Autodesk Inventor part; units mm, degrees
ref_plane "YZ Plane" through (0, 0, 0) normal (1, 0, 0) x (0, 1, 0)
ref_plane "XZ Plane" through (0, 0, 0) normal (0, 1, 0) x (-1, 0, 0)
ref_plane "XY Plane" through (0, 0, 0) normal (0, 0, 1) x (1, 0, 0)
ref_plane "Work Plane1" through (0, 0, 0) normal (0, 0, 1) x (1, 0, 0)
sketch "Sketch1" plane through (0, 0, 0) normal (0, 0, 1) x (1, 0, 0)
  circle A0 centre (114.3836, 12.2466) radius 10
  circle A1 centre (114.3836, 12.2466) radius 10
  line L0 (114.3836, 12.2466) -> (76.8836, 12.2466)
  line L1 (124.7866, -536.2038) -> (-25.2134, -536.2038)
  line L2 (114.3836, 12.2466) -> (114.3836, -536.2038)
  line L3 (76.8836, 12.2466) -> (76.8836, 52.1676)
  line L4 (76.8836, 52.1676) -> (226.8836, 52.1676)
  line L5 (226.8836, 52.1676) -> (226.8836, -17.8324)
  line L6 (226.8836, -17.8324) -> (76.8836, -17.8324)
  line L7 (76.8836, -17.8324) -> (76.8836, 12.2466)
  circle A2 centre (114.3836, 12.2466) radius 10
  line L8 (151.8836, 52.1676) -> (151.8836, -17.8324)
  circle A3 centre (189.3836, 12.2466) radius 10
  line L9 (76.8836, 52.1676) -> (76.8836, 42.1676)
  line L10 (76.8836, 42.1676) -> (226.8836, 42.1676)
  line L11 (226.8836, 52.1676) -> (76.8836, 52.1676)
  line L12 (76.8836, 52.1676) -> (76.8836, 42.1676)
  line L13 (76.8836, 42.1676) -> (226.8836, 42.1676)
  line L14 (226.8836, 42.1676) -> (226.8836, 52.1676)
  point P0 (0, 0)
  dimension "d0" = 37.5
  dimension "d1" = 548.4504
  dimension "d2" = 39.921
  dimension "d3" = 150
  dimension "d4" = 70
  dimension "d5" = 10
  dimension "d6" = 150
extrude "Extrusion1" add sketch "Sketch1" along normal blind 5 contours A0 L0 L3 L10 L8 L6 L2 | A0 L2 L6 L7 L0 | L3 L4 L8 L10 | L8 L10 L5 L6 | L8 L4 L5 L10
sketch "Sketch3" plane through (0, 0, 0) normal (0, 0, -1) x (-1, 0, 0)
  line L0 (-226.8836, 52.1676) -> (-76.8836, 52.1676)
  line L1 (-76.8836, 42.1676) -> (-226.8836, 42.1676)
  line L2 (-226.8836, 52.1676) -> (-76.8836, 52.1676)
  line L3 (-76.8836, 52.1676) -> (-76.8836, 42.1676)
  line L4 (-76.8836, 42.1676) -> (-226.8836, 42.1676)
  line L5 (-226.8836, 42.1676) -> (-226.8836, 52.1676)
  point P0 (0, 0)
extrude "Extrusion2" add sketch "Sketch3" along normal blind 80
sketch "Sketch4" plane through (0, 0, -80) normal (0, 0, -1) x (-1, 0, 0)
  line L0 (-226.8836, 52.1676) -> (-76.8836, 52.1676)
  line L1 (-76.8836, -17.8324) -> (-226.8836, -17.8324)
  line L2 (-226.8836, 52.1676) -> (-76.8836, 52.1676)
  line L3 (-76.8836, 52.1676) -> (-76.8836, -17.8324)
  line L4 (-76.8836, -17.8324) -> (-226.8836, -17.8324)
  line L5 (-226.8836, -17.8324) -> (-226.8836, 52.1676)
  point P0 (0, 0)
  point P1 (-76.8836, 52.1676)
extrude "Extrusion3" add sketch "Sketch4" along normal blind 5
sketch "Sketch6" plane through (0, 0, -85) normal (0, 0, -1) x (-1, 0, 0)
  line L0 (-98.3957, 24.2628) -> (62.6208, -189.9747)
  arc A0 (-98.3957, 24.2628) -> (-130.3715, 0.2304) centre (-114.3836, 12.2466) ccw
  line L1 (30.6451, -214.007) -> (-130.3715, 0.2304)
  arc A1 (30.6451, -214.007) -> (62.6208, -189.9747) centre (46.6329, -201.9908) ccw
  circle A2 centre (46.6329, -201.9908) radius 9.25
  circle A3 centre (-114.3836, 12.2466) radius 10
  circle A4 centre (-189.3836, 12.2466) radius 10
  point P0 (0, 0)
extrude "Extrusion4" cut sketch "Sketch6" against normal blind 10 contours A3 | A4
sketch "Sketch8" plane through (76.8836, 52.1676, 5) normal (0, 1, 0) x (1, 0, 0)
  line L0 (0, 0) -> (0, 90)
  line L1 (150, 0) -> (0, 0)
  line L2 (150, 90) -> (150, 0)
  line L3 (0, 90) -> (150, 90)
  point P0 (-76.8836, 5)
extrude "Extrusion6" add sketch "Sketch8" along normal blind 0.079
properties part number "korona"
Geometry: final body of the model. Coordinates: model frame, mm. A direction names the side the tool comes from. Round coordinates to 2 decimals unless told otherwise and drop trailing zeros. Write each loop counter-clockwise with the first axis right and the second up, starting at its lowest first coordinate (ties: lowest second). Pieces come first, ordered by that corner, then holes.
Item 1: Section query A-A (y = -4). Return loops of the section in (x, z).
Item 2: Material intervals for L1, parallel to Z at x = 96.5, y = 39.5; L2, parallel to Y at x = 131.5, z = -17; L3, parallel to Y at x = 108, z = 0.5, sorted ascending.
Item 3: Pin query (flat end, axial travel): P1, Ø5, axis at x = 118.5, z = -64, coming from the -Y side. Return the tip coordinate at first contact, or that it passes through.
Item 4: Section query D-D (x = 189). Return loops of the section in (y, z), plus the area to 3 significant figures.
Item 5: Set-up query: faces 4 (the face through (151, 42.168, -39)), 5 (the face through (180.146, 8.417, -82.535)). Return all of +Z, -Z, +X, -X, +Y, -Y with unobstructed straight access to the full face (end or side cutting, diameter ignored); none if empty.
Item 6: Section query B-B (y = 6.5). Return loops of the section in (x, z).
Item 7: Section query C-C (x = 87.5). Return loops of the section in (y, z).
Item 8: Mould query, pull axis Y, two halves, no side actions, for faces 1 (the face through (153, 13, -80)), 2 (the face through (151, -17.832, -82)), 3 (the face through (104.393, 11.807, 2.465)). Classes: +Y half, -Y half, draft (parallel to the pull), parting line (faces both ways), or undercut.
Completed:
1. outline: (76.88, -85) - (226.88, -85) - (226.88, -80) - (76.88, -80) - close; (76.88, 0) - (226.88, 0) - (226.88, 5) - (76.88, 5) - close
2. L1: z = -85 to -80, 0 to 5
2. L2: y = 42.17 to 52.25
2. L3: y = -17.83 to 4.55, 19.94 to 52.25
3. P1: stops at y = 42.17
4. outline: (-17.83, -85) - (2.25, -85) - (2.25, -80) - (-17.83, -80) - close; (-17.83, 0) - (2.25, 0) - (2.25, 5) - (-17.83, 5) - close; (22.24, -85) - (52.25, -85) - (52.25, 5) - (22.24, 5) - (22.24, 0) - (42.17, 0) - (42.17, -80) - (22.24, -80) - close
4. area: 1,310 mm2
5. face 4: +X, -X, -Y
5. face 5: +Z, -Z
6. outline: (76.88, -85) - (106.2, -85) - (106.2, -80) - (76.88, -80) - close; (76.88, 0) - (106.2, 0) - (106.2, 5) - (76.88, 5) - close; (122.57, -85) - (181.2, -85) - (181.2, -80) - (122.57, -80) - close; (122.57, 0) - (181.2, 0) - (181.2, 5) - (122.57, 5) - close; (197.57, -85) - (226.88, -85) - (226.88, -80) - (197.57, -80) - close; (197.57, 0) - (226.88, 0) - (226.88, 5) - (197.57, 5) - close
7. outline: (-17.83, -85) - (52.25, -85) - (52.25, 5) - (-17.83, 5) - (-17.83, 0) - (42.17, 0) - (42.17, -80) - (-17.83, -80) - close
8. face 1: draft
8. face 2: -Y half
8. face 3: undercut
